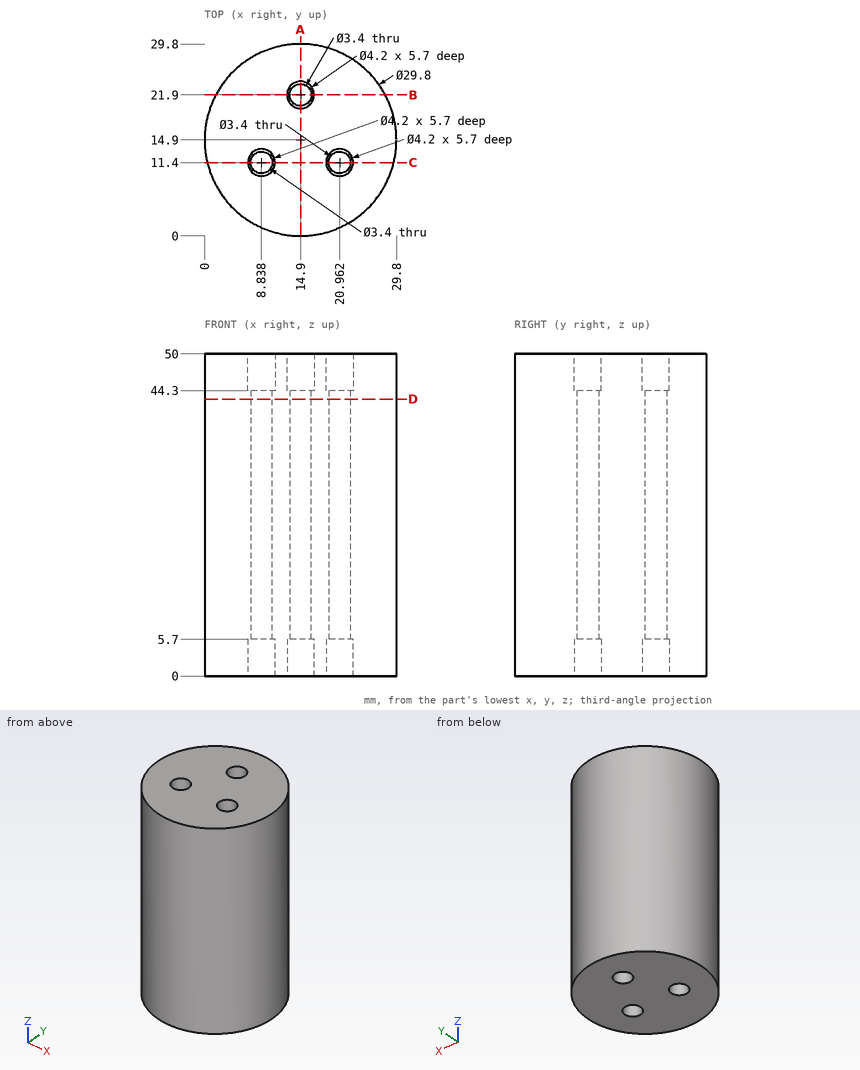
Here's the drawing with two shaded views (mm, measured from the low corner). I have some questions. Coordinates: 2 decimals unless noted, no trailing zeros. Order: outer loops, then holes, each group sorted by start corner. A loop starts at its lowest first (then second) coordinate and runs counter-clockwise, first axis right, second up. Notation, with made-up numbers: (80.5, 69) - (112.5, 69) arc R21 ccw to (112.5, 90) - close; hole circle Ø1 at (37.25, 71). An arc over 180 degrees is marked (long way). Use CSV: the item, a comma, the result in double quotes. Start each with the question number.
1. Suppose I cut it at A-A on x = 14.9. List the corners of the cut face in (y, z) for me, then the cut area to 3 significant figures.
2. Suppose I cut it at B-B on y = 21.9. List the corners of the cut face in (x, z) for me, then the cut area to 3 significant figures.
3. Suppose I cut it at C-C on y = 11.4. List the corners of the cut face in (x, z) for me, then the cut area to 3 significant figures.
4. Please list where these lines run through material, in increasing order: line 1 (X direction, y = 10, z = 3); line 2 (X direction, y = 11.4, z = 15); line 3 (Z direction, x = 19.25, y = 12.5). Write a range as from..to.
5. I'm going to push flat-ended pins straight in: pin 1 (4 mm diameter, centred on x = 20.96, y = 11.4, fed in from -Z); pin 2 (4 mm diameter, centred on x = 14.9, y = 21.9, fed in from +Z); pin 3 (2 mm diameter, centred on x = 14.9, y = 21.9, fed in from +Z); pin 4 (8 mm diameter, centred on x = 20, z = 9, fed in from -Y). Where does each tip first touch, or does it pass through?
6. Suppose I cut it at D-D on z = 43. List the corners of the cut face in (x, y) for me, then the cut area to 3 significant figures.
Output:
1,outline,"(0, 0) - (19.8, 0) - (19.8, 5.7) - (20.2, 5.7) - (20.2, 44.3) - (19.8, 44.3) - (19.8, 50) - (0, 50) - close; (23.6, 5.7) - (24, 5.7) - (24, 0) - (29.8, 0) - (29.8, 50) - (24, 50) - (24, 44.3) - (23.6, 44.3) - close"
1,area,"1,310 mm2"
2,outline,"(1.75, 0) - (12.8, 0) - (12.8, 5.7) - (13.2, 5.7) - (13.2, 44.3) - (12.8, 44.3) - (12.8, 50) - (1.75, 50) - close; (16.6, 5.7) - (17, 5.7) - (17, 0) - (28.05, 0) - (28.05, 50) - (17, 50) - (17, 44.3) - (16.6, 44.3) - close"
2,area,"1,140 mm2"
3,outline,"(0.42, 0) - (6.74, 0) - (6.74, 5.7) - (7.14, 5.7) - (7.14, 44.3) - (6.74, 44.3) - (6.74, 50) - (0.42, 50) - close; (10.54, 5.7) - (10.94, 5.7) - (10.94, 0) - (18.86, 0) - (18.86, 5.7) - (19.26, 5.7) - (19.26, 44.3) - (18.86, 44.3) - (18.86, 50) - (10.94, 50) - (10.94, 44.3) - (10.54, 44.3) - close; (22.66, 5.7) - (23.06, 5.7) - (23.06, 0) - (29.38, 0) - (29.38, 50) - (23.06, 50) - (23.06, 44.3) - (22.66, 44.3) - close"
3,area,"1,090 mm2"
4,line 1,"x = 0.83..7.27, 10.4..19.4, 22.53..28.97"
4,line 2,"x = 0.42..7.14, 10.54..19.26, 22.66..29.38"
4,line 3,"z = 5.7..44.3"
5,pin 1,"stops at z = 5.7"
5,pin 2,"stops at z = 44.3"
5,pin 3,"passes through"
5,pin 4,"stops at y = 0.04"
6,outline,"circle Ø29.8 at (14.9, 14.9); hole circle Ø3.4 at (8.84, 11.4); hole circle Ø3.4 at (14.9, 21.9); hole circle Ø3.4 at (20.96, 11.4)"
6,area,"670 mm2"
